The listing builds one solid part. Answer for the finished solid, in the listing's coordinates (mm). A direction names the side the tool comes from. Round coordinates to 2 decimals unless told otherwise and drop trailing zeros. Order: outer loops, then holes, each group sorted by start corner. A loop starts at its lowest first (then second) coordinate and runs counter-clockwise, first axis right, second up. Notation, with made-up numbers: (-20.5, -5) - (8.5, -5) arc R8 cw to (8.5, 2) - close; hole circle Ø3 at (44, 49). An arc over 180 degrees is marked (long way). One line per item, written item: value. Start each with the question number.
1. Section A-A, the plane x = 0 is taken. Give the vertices of the cut face in (y, z), then the cut area to 4 significant figures.
2. Section D-D, the plane z = 12.5 is taken. Give the vertices of the cut face in (x, y), then the cut area to 3 significant figures.
3. For a pull along Y with two mould halves and no side action, classify faces 4 (the cylindrical face through (-9.325, -49.464, 5.07)), 5 (the flat face through (-0.056, -59.72, 12.535)), 6 (the flat face through (-12.5, -60, -6)) as released by +Y, released by -Y, zero draft, split by the parting line, or undercut.
4. Section C-C, the plane y = -70 is taken. Give the vertices of the cut face in (x, z).
5. Flat-ended cylindrical pins translate along their axes: P1, Ø1.5, axis at y = -49, z = -2, coming from the -X side; P2, Ø4, axis at x = 9, y = -48, coming from the +Z side; P3, Ø4, axis at x = 9, y = -59, coming from the -Z side. Find the tip coordinate at first contact, or state that the pin passes through.
6. Straight lines are drawn through the part: line 1 (Y direction, x = -9, z = 7.75); line 2 (X direction, y = -70, z = 7); line 3 (X direction, y = -75, z = -11.5). For each, find the intervals that lie inside material, in ascending order.
7. A tool of negligible diameter and unlimited length cuts with its end or side. For faces 1 (the flat face through (-22.5, -60, -6)), 2 (the flat face through (28, 17, 4)), 3 (the cylindrical face through (-31, 9.76, 5.48)), from which of +Z, -Z, +X, -X, +Y, -Y can it reach the whole face along a straight path? Write none if from no direction.
8. Section B-B, the plane z = -2.5 is taken. Give the vertices of the cut face in (x, y).
from build123d import *

# Parameters (mm, degrees)
SKETCH1_R               = 37.5
SKETCH1_R_2             = 29.5
BOSS_EXTRUDE1_DEPTH     = 15
SKETCH2_R               = 32.5
SKETCH2_R_2             = 27.5
CUT_EXTRUDE1_DEPTH      = 7
SKETCH9_R               = 1
CUT_EXTRUDE5_DEPTH      = 15
SKETCH10_R              = 37.5
CUT_EXTRUDE6_DEPTH      = 4
CUT_EXTRUDE7_DEPTH      = 35
CUT_EXTRUDE7_DEPTH_BACK = 35
SKETCH12_W              = 10
SKETCH12_H              = 40
CUT_EXTRUDE8_DEPTH      = 5
SKETCH13_R              = 1.5
SKETCH13_R_2            = 1.68215716
CUT_EXTRUDE9_DEPTH      = 10
SKETCH14_W              = 10
SKETCH14_H              = 40
BOSS_EXTRUDE2_DEPTH     = 12.5


with BuildPart() as part:
    # Sketch1 → Boss-Extrude1 (new body)
    # profile 1 of 2: a face of its own
    with BuildSketch(Plane.XY):
        Circle(SKETCH1_R)
        Circle(SKETCH1_R_2, mode=Mode.SUBTRACT)
    # profile 2 of 2: a face of its own
    with BuildSketch(Plane.XY):
        with BuildLine():
            Line((-22.5, -80), (22.5, -80))
            Line((22.5, -80), (36.796608813, -7.229078771))
            ThreePointArc((36.796608813, -7.229078771), (0, -37.5), (-36.796608813, -7.229078771))
            Line((-36.796608813, -7.229078771), (-22.5, -80))
        make_face()
    extrude(amount=BOSS_EXTRUDE1_DEPTH)

    # Sketch2 → Cut-Extrude1 (cut)
    with BuildSketch(Plane(origin=(0, 0, 0), x_dir=(-1, 0, 0), z_dir=(0, 0, -1))):
        Circle(SKETCH2_R)
        Circle(SKETCH2_R_2, mode=Mode.SUBTRACT)
    extrude(amount=-CUT_EXTRUDE1_DEPTH, mode=Mode.SUBTRACT)

    # Sketch9 → Cut-Extrude5 (cut)
    with BuildSketch(Plane.XY.offset(15)):
        with Locations((17, 29.444863729)):
            Circle(SKETCH9_R)
        with Locations((34, 0)):
            Circle(SKETCH9_R)
        with Locations((17, -29.444863729)):
            Circle(SKETCH9_R)
        with Locations((-17, -29.444863729)):
            Circle(SKETCH9_R)
        with Locations((-34, 0)):
            Circle(SKETCH9_R)
        with Locations((-17, 29.444863729)):
            Circle(SKETCH9_R)
    extrude(amount=-CUT_EXTRUDE5_DEPTH, mode=Mode.SUBTRACT)

    # Sketch10 → Cut-Extrude6 (cut)
    with BuildSketch(Plane(origin=(0, 0, 0), x_dir=(-1, 0, 0), z_dir=(0, 0, -1))):
        Circle(SKETCH10_R)
    extrude(amount=-CUT_EXTRUDE6_DEPTH, mode=Mode.SUBTRACT)

    # Sketch11 → Cut-Extrude7 (cut, two sides: drawn at the far end of the back side and taken through both)
    with BuildSketch(Plane(origin=(0, 0, 0), x_dir=(0, 0, -1), z_dir=(1, 0, 0)).offset(-CUT_EXTRUDE7_DEPTH_BACK)):
        Polygon((-15, -80), (-15, -40), (-10, -80), align=None)
    extrude(amount=CUT_EXTRUDE7_DEPTH + CUT_EXTRUDE7_DEPTH_BACK, mode=Mode.SUBTRACT)

    # Sketch12 → Cut-Extrude8 (cut)
    with BuildSketch(Plane.XY.offset(15)):
        with Locations((-9, -60)):
            Rectangle(SKETCH12_W, SKETCH12_H)
        with Locations((9, -60)):
            Rectangle(SKETCH12_W, SKETCH12_H)
    extrude(amount=-CUT_EXTRUDE8_DEPTH, mode=Mode.SUBTRACT)

    # Sketch13 → Cut-Extrude9 (cut)
    with BuildSketch(Plane.XY.offset(10)):
        with Locations((-9, -48)):
            Circle(SKETCH13_R)
        with Locations((-9, -59)):
            Circle(SKETCH13_R)
        with Locations((-9, -70)):
            Circle(SKETCH13_R_2)
        with Locations((9, -70)):
            Circle(SKETCH13_R)
        with Locations((9, -59)):
            Circle(SKETCH13_R)
        with Locations((9, -48)):
            Circle(SKETCH13_R)
    extrude(amount=-CUT_EXTRUDE9_DEPTH, mode=Mode.SUBTRACT)

    # Sketch14 → Boss-Extrude2 (add)
    with BuildSketch(Plane(origin=(0, 0, 0), x_dir=(-1, 0, 0), z_dir=(0, 0, -1))):
        with Locations((-17.5, -60)):
            Rectangle(SKETCH14_W, SKETCH14_H)
        with Locations((17.5, -60)):
            Rectangle(SKETCH14_W, SKETCH14_H)
    extrude(amount=BOSS_EXTRUDE2_DEPTH)


solid = part.part
Answer list:
1. outline: (-80, 0) - (-37.5, 0) - (-37.5, 4) - (-32.5, 4) - (-32.5, 7) - (-29.5, 7) - (-29.5, 15) - (-40, 15) - (-80, 10) - close; (29.5, 7) - (32.5, 7) - (32.5, 4) - (37.5, 4) - (37.5, 15) - (29.5, 15) - close
1. area: 695.5 mm²
2. outline: (-36.8, -7.23) - (-26.43, -60) - (-14, -60) - (-14, -40) - (-4, -40) - (-4, -60) - (4, -60) - (4, -40) - (14, -40) - (14, -60) - (26.43, -60) - (36.8, -7.23) arc R37.5 ccw (long way) to start; hole circle Ø2 at (-34, 0); hole circle Ø59 at (0, 0); hole circle Ø2 at (-17, -29.44); hole circle Ø2 at (-17, 29.44); hole circle Ø2 at (17, -29.44); hole circle Ø2 at (17, 29.44); hole circle Ø2 at (34, 0)
2. area: 2,930 mm²
3. face 4: undercut
3. face 5: released by -Y
3. face 6: zero draft
4. outline: (-24.46, 0) - (-22.5, 0) - (-22.5, -12.5) - (-12.5, -12.5) - (-12.5, 0) - (-10.68, 0) - (-10.68, 10) - (-14, 10) - (-14, 11.25) - (-24.46, 11.25) - close; (-7.32, 0) - (7.5, 0) - (7.5, 10) - (4, 10) - (4, 11.25) - (-4, 11.25) - (-4, 10) - (-7.32, 10) - close; (10.5, 0) - (12.5, 0) - (12.5, -12.5) - (22.5, -12.5) - (22.5, 0) - (24.46, 0) - (24.46, 11.25) - (14, 11.25) - (14, 10) - (10.5, 10) - close
5. P1: stops at x = -22.5
5. P2: stops at z = 10
5. P3: stops at z = 0
6. line 1: y = -80 to -71.68, -68.32 to -60.5, -57.5 to -49.5, -46.5 to -28.09, 28.09 to 36.4
6. line 2: x = -24.46 to -10.68, -7.32 to 7.5, 10.5 to 24.46
6. line 3: x = -22.5 to -12.5, 12.5 to 22.5
7. face 1: -Z, -X, +Y, -Y
7. face 2: -Z, +Y
7. face 3: -Z
8. outline: (-22.5, -80) - (-12.5, -80) - (-12.5, -40) - (-22.5, -40) - close; (12.5, -80) - (22.5, -80) - (22.5, -40) - (12.5, -40) - close
